Autodesk Inventor part; units mm, degrees
ref_plane "YZ Plane" through (0, 0, 0) normal (1, 0, 0) x (0, 1, 0)
ref_plane "XZ Plane" through (0, 0, 0) normal (0, 1, 0) x (-1, 0, 0)
ref_plane "XY Plane" through (0, 0, 0) normal (0, 0, 1) x (1, 0, 0)
sketch "Sketch1" plane through (0, 0, 0) normal (0, 0, 1) x (1, 0, 0)
  line L0 (2.667, 0) -> (19.05, 0)
  line L1 (19.05, 0) -> (19.05, 3.81)
  line L2 (19.05, 3.81) -> (3.937, 3.81)
  line L3 (3.937, 3.81) -> (3.937, 11.43)
  line L4 (3.937, 11.43) -> (2.667, 11.43)
  line L5 (2.667, 11.43) -> (2.667, 0)
  line L6 (0, 25.5419) -> (0, -2.7317)
  point P0 (0, 0)
  dimension "d11" = 19.05
  dimension "d12" = 3.81
  dimension "d13" = 1.27
  dimension "d15" = 2.667
  dimension "d16" = 7.62
revolve "Revolution1" add sketch "Sketch1" angle 360 about axis through (0, 25.5419, 0) along (0, -1, 0)
fillet "Fillet1" radius 6.35 1 edges at (-3.937, 3.81, 0)
fillet "Fillet2" radius 1.905 2 edges at (-19.05, 3.81, 0) (-19.05, 0, 0)
properties part number "Front Wheel"
The listing builds one solid part. Answer for the finished solid, in the listing's coordinates (mm). A direction names the side the tool comes from. Round coordinates to 2 decimals unless told otherwise and drop trailing zeros. Write each loop counter-clockwise with the first axis right and the second up, starting at its lowest first coordinate (ties: lowest second). Pieces come first, ordered by that corner, then holes. Notation, with made-up numbers: (3.25, -32.75) -> (42.25, -32.75) arc R21 ccw to (42.25, -12.75) -> close; hole circle Ø8 at (19.25, 4). An arc over 180 degrees is marked (long way). Use CSV: the item, a comma, the result in double quotes. Start each with the question number.
(1) Which of the six approach directions +Z, -Z, +X, -X, +Y, -Y give full straight-line access (tool end or side, diameter ignored) to faces 1 (the face through (4, 0, 0)), 2 (the face through (7.4, 3.81, -7.4))?
(2) Each of these flat-tipped pins is pushed along its axis until it touches: pin 1 (3 mm diameter, centred on y = 4, z = -8, fed in from -X); pin 2 (1.5 mm diameter, centred on x = 12, y = 4, fed in from +Z); pin 3 (4 mm diameter, centred on x = -8.5, z = 2.5, fed in from +Y). Where does it stop, or does it pass through?
(3) The mould has two halves that part along Z. Classify faces 3 (the face through (-0.853, 10.804, 3.843)), 4 (the face through (1.231, 5.635, -2.366)), 5 (the face through (1, 11.43, -3)): released by +Z, released by -Z, zero draft, split by the parting line, or undercut.
(4) Section C-C on y = 5.5 is taken. Give the vertices of the cut face in (x, z).
(5) Consider L1, parallel to Z at x = 0, y = 6; L2, parallel to Y at x = 10, z = 13; L3, parallel to Z at x = 0, y = 5.5. Determine where each line is inside the solid, lowest interval first. Write a range as from..to.
A:
1,face 1,"+Z, -Z, +X, -X, -Y"
1,face 2,"+Y"
2,pin 1,"stops at x = -17.44"
2,pin 2,"stops at z = 14.24"
2,pin 3,"stops at y = 4.81"
3,face 3,"split by the parting line"
3,face 4,"undercut"
3,face 5,"zero draft"
4,outline,"circle Ø11.95 at (0, 0); hole circle Ø5.33 at (0, 0)"
5,L1,"z = -5.49..-2.67, 2.67..5.49"
5,L2,"y = 0..3.81"
5,L3,"z = -5.97..-2.67, 2.67..5.97"
